```python
from build123d import *

# Parameters (mm, degrees)
SKETCH2_R          = 5
CUT_EXTRUDE1_DEPTH = 34


with BuildPart() as part:
    # Sketch1 → Revolve1 (revolve)
    with BuildSketch(Plane.XY, mode=Mode.PRIVATE) as revolve1_sk:
        Polygon((0, 0), (0, 22), (0, 23), (-27.5, 23), (-27.5, 22), (-25, 22), (-25, 0), (-27.5, 0), (-27.5, -1), (-19, -1), (-19, -9), (0, -9), (0, -1), align=None)
    revolve(revolve1_sk.sketch.rotate(Axis((0, 0, 0), (0, 1, 0)), 270), axis=Axis((0, 0, 0), (0, 1, 0)))

    # Sketch2 → Cut-Extrude1 (cut)
    with BuildSketch(Plane(origin=(0, 23, 0), x_dir=(1, 0, 0), z_dir=(0, 1, 0))):
        with Locations(Location((0, 0, 0), (0, 0, 270))):
            Circle(SKETCH2_R)
    extrude(amount=-CUT_EXTRUDE1_DEPTH, mode=Mode.SUBTRACT)


solid = part.part
```
Read the model definition and answer for the solid it produces. Units are mm, in the model's axes. A direction names the side the tool comes from. Give positions to 0.01 mm unless a question says otherwise; leave off trailing zeros. Loops run counter-clockwise (first coordinate to the right, second up) from the corner with the lowest first, then second, coordinate; pieces in that order, holes last.
Item 1: The mould has two halves that part along Y. Classify faces 4 (the flat face through (4, -9, -4)), 5 (the cylindrical face through (-7.509, 10.846, -23.846)), 6 (the cylindrical face through (-4.88, 7.22, -1.08)): released by +Y, released by -Y, zero draft, split by the parting line, or undercut.
Item 2: Find the intervals of material crossed by line 1 along X through (y, z) = (3, 0); line 2 along X through (y, z) = (-2, 0); line 3 along Y through (x, z) = (-23, -11), in increasing order.
Item 3: The part is cut by section D-D (y = 20.5). Write down the section's boundary in (x, z), and give its area (3 significant figures).
Item 4: The part is cut by section A-A (x = 0). Write down the section's boundary in (y, z), and give its area (3 significant figures).
Item 5: The part is cut by section B-B (z = 0). Write down the section's boundary in (x, y).
Item 6: For faces 1 (the flat face through (6, 23, 0)), 2 (the flat face through (-19, -1, -6)), 3 (the flat face through (22.3, 22, -12.1)), determine the directions among +Z, -Z, +X, -X, +Y, -Y from which every point of the face is accessible in a straight line to the end or side of a thin tool.
Item 7: The part is cut by section C-C (x = -21.5). Write down the section's boundary in (y, z).
Item 8: Each of these flat-tipped pins is pushed along its axis until it touches: pin 1 Ø4 at (y, z) = (17, 6) entering from +X; pin 2 Ø4 at (y, z) = (10, 6.5) entering from +X; pin 3 Ø3 at (y, z) = (0, -4.5) entering from -X. Where does it stop, or does it pass through?
Taken from the geometry:
1. face 4: released by -Y
1. face 5: undercut
1. face 6: zero draft
2. line 1: x = -25 to -5, 5 to 25
2. line 2: x = -19 to -5, 5 to 19
2. line 3: y = -1 to 0, 22 to 23
3. outline: circle Ø50 at (0, 0); hole circle Ø10 at (0, 0)
3. area: 1,880 mm2
4. outline: (-9, -19) - (-1, -19) - (-1, -27.5) - (0, -27.5) - (0, -25) - (22, -25) - (22, -27.5) - (23, -27.5) - (23, -5) - (-9, -5) - close; (-9, 5) - (23, 5) - (23, 27.5) - (22, 27.5) - (22, 25) - (0, 25) - (0, 27.5) - (-1, 27.5) - (-1, 19) - (-9, 19) - close
4. area: 1,190 mm2
5. outline: (-27.5, -1) - (-19, -1) - (-19, -9) - (-5, -9) - (-5, 23) - (-27.5, 23) - (-27.5, 22) - (-25, 22) - (-25, 0) - (-27.5, 0) - close; (5, -9) - (19, -9) - (19, -1) - (27.5, -1) - (27.5, 0) - (25, 0) - (25, 22) - (27.5, 22) - (27.5, 23) - (5, 23) - close
6. face 1: +Z, -Z, +X, -X, +Y
6. face 2: -Y
6. face 3: none
7. outline: (-1, -17.15) - (0, -17.15) - (0, -12.76) - (22, -12.76) - (22, -17.15) - (23, -17.15) - (23, 17.15) - (22, 17.15) - (22, 12.76) - (0, 12.76) - (0, 17.15) - (-1, 17.15) - close
8. pin 1: stops at x = 24.68
8. pin 2: stops at x = 24.59
8. pin 3: stops at x = -27.34
